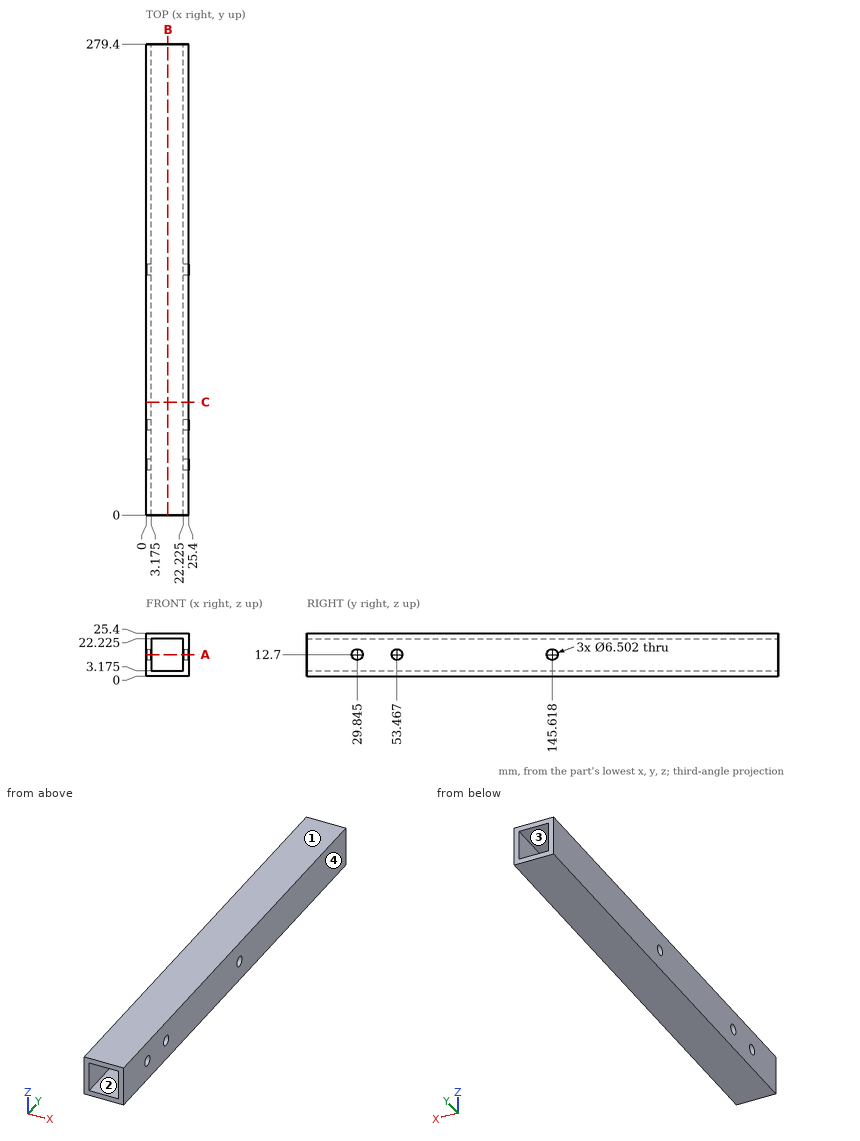
For this review, use the dimensioned drawing (mm, ordinates from the lowest corner) and the shaded views. Round coordinates to 2 decimals unless told otherwise and drop trailing zeros. Order: outer loops, then holes, each group sorted by start corner. A loop starts at its lowest first (then second) coordinate and runs counter-clockwise, first axis right, second up. Notation, with made-up numbers: (-40, 72.25) -> (-36, 72.25) arc R33 cw to (-36, 109.25) -> close; hole circle Ø9 at (78, 52). An arc over 180 degrees is marked (long way). Put each result on its own line as item: value.
Q1. Add section B-B on x = 13. Write out the cut boundary in (y, z) (1 decimal).
Check result:
outline: (0, 0) -> (279.4, 0) -> (279.4, 3.2) -> (0, 3.2) -> close; (0, 22.2) -> (279.4, 22.2) -> (279.4, 25.4) -> (0, 25.4) -> close
Q2. Add section A-A on z = 12.7. State how many separate pieces and enclosed holes the cut face has, plus the area to 3 significant figures.
Check result:
separate pieces: 8
enclosed holes: 0
area: 1,650 mm2
Q3. Mouldability with a two-part tool opening along Z and no side actions: class the marked faces 1, 2, 3 and 4 as pulls with the +Z half, pulls with the -Z half, needs draft (parallel to the pull), parting line crosses it, or undercut.
Check result:
face 1: pulls with the +Z half
face 2: undercut
face 3: undercut
face 4: needs draft
Q4. Add section C-C on y = 67. Write out the cut boundary in (x, z) (1 decimal).
Check result:
outline: (0, 0) -> (25.4, 0) -> (25.4, 25.4) -> (0, 25.4) -> close; hole (3.2, 3.2) -> (22.2, 3.2) -> (22.2, 22.2) -> (3.2, 22.2) -> close
Q5. For probe 1 along Y at (x, z) = (2.3, 12.7) (1 decimal); probe 2 along Z at (x, y) = (7.5, 94.5) (1 decimal), list the stretches that pass through material, from the lowest coordinate up. Write a range as [from, to].
Check result:
probe 1: [0, 26.6], [33.1, 50.2], [56.7, 142.4], [148.9, 279.4]
probe 2: [0, 3.2], [22.2, 25.4]
